For this review, take the finished solid that the model builds, in its own axes (mm). A direction names the side the tool comes from. Coordinates: 2 decimals unless noted, no trailing zeros. Loops run counter-clockwise (first coordinate to the right, second up) from the corner with the lowest first, then second, coordinate; pieces in that order, holes last.
1. Clearance check with flat-ended pins moving along their axes: P1, Ø4, axis at x = 7, z = 18.5, coming from the +Y side; P2, Ø4, axis at y = 8.5, z = 13, coming from the -X side; P3, Ø1, axis at y = 11, z = 27.5, coming from the -X side; P4, Ø12, axis at x = 0, y = 0, coming from the +Z side. State where each tip first meets the part, or that it passes through.
2. To check wall thickness, follow probe 1 along X at (y, z) = (0.5, 30); probe 2 along Y at (x, z) = (0, 9). State the ranges of each line that lie inside material, in increasing order.
3. Mouldability with a two-part tool opening along Y and no side actions: class faces 4 (the face through (0, -18.371, 27)), 5 (the face through (5, -7, 11.906)), 6 (the face through (8, -15, 21.828)) as pulls with the +Y half, pulls with the -Y half, needs draft (parallel to the pull), parting line crosses it, or undercut.
4. Take a section at A-A, the plane y = 0. State the section outline as (x, z) points.
5. Take a section at C-C, the plane z = 25.5. State the section outline as (x, y) points.
6. Machinability: for faces 1 (the face through (-3.62, -16.303, 10.761)), 2 (the face through (4.923, -9.464, 21.689)), 3 (the face through (12.91, -13.07, 26.72)), which of the approach directions +Z, -Z, +X, -X, +Y, -Y give a long, thin tool a straight path to every point of the face, cutting with its end or side? Answer none if there is none.
7. Take a section at D-D, the plane x = 15. State the section outline as (y, z) points, then the cut area to 3 significant figures.
```python
from build123d import *

# Parameters (mm, degrees)
OBJ1_R     = 10.668
OBJ1_DEPTH = 19.84375
OBJ2     = 7.6454
OBJ3 = 31.75
BOX001_W               = 36.7411
BOX001_H               = 36.7411
BOX001_DEPTH           = 9.921875
BOX001_PLACEMENT_ANGLE = 45
BOX_W                  = 36.7411
BOX_H                  = 36.7411
BOX_DEPTH              = 9.921875
OBJ4        = 16.7005
OBJ5    = 31.75


with BuildPart() as obj1:
    # obj1 → obj1 (new body)
    with BuildSketch(Plane.XY.offset(11.90625)):
        Circle(OBJ1_R)
    extrude(amount=OBJ1_DEPTH)


with BuildPart() as cone:
    # Cone → Cone (revolve)
    with BuildSketch(Plane.XZ):
        Polygon((0, 0), (12.17295, 0), (7.6454, 5.953125), (0, 5.953125), align=None)
    revolve(axis=Axis((0, 0, 0), (0, 0, 1)))


with BuildPart() as fusion001:
    with BuildSketch(Plane.XY):
        Circle(OBJ2)
    extrude(amount=OBJ3)

    # Fusion001: union obj1, Cone
    add(obj1.part)
    add(cone.part)


with BuildPart() as box001:
    # Box001 → Box001 (new body)
    with BuildSketch(Plane.XY):
        with Locations((18.37055, 18.37055)):
            Rectangle(BOX001_W, BOX001_H)
    extrude(amount=BOX001_DEPTH)


with BuildPart() as box001_1:
    # Box001 placement: moved
    add(box001.part.moved(Location((0, -25.979881, 0))).rotate(Axis((0, -25.979881, 0), (0, 0, 1)), BOX001_PLACEMENT_ANGLE))


with BuildPart() as common:
    # Box → Box (new body)
    with BuildSketch(Plane(origin=(-18.37055, -18.37055, 0), x_dir=(1, 0, 0), z_dir=(0, 0, 1))):
        with Locations((18.37055, 18.37055)):
            Rectangle(BOX_W, BOX_H)
    extrude(amount=BOX_DEPTH)

    # Common: intersect Box001
    add(box001_1.part, mode=Mode.INTERSECT)


with BuildPart() as common_1:
    # Common placement: moved
    add(common.part.moved(Location((0, 0, 21.828125))))


with BuildPart() as cut:
    with BuildSketch(Plane.XY):
        Circle(OBJ4)
    extrude(amount=OBJ5)

    # Fusion: union Common
    add(common_1.part)

    # Cut: cut Fusion001
    add(fusion001.part, mode=Mode.SUBTRACT)


solid = cut.part
```
Results list:
1. P1: stops at y = 15.93
1. P2: stops at x = -15.38
1. P3: stops at x = -15.48
1. P4: passes through
2. probe 1: x = -18.37 to -10.66, 10.66 to 18.37
2. probe 2: y = -16.7 to -7.65, 7.65 to 16.7
3. face 4: pulls with the -Y half
3. face 5: undercut
3. face 6: needs draft
4. outline: (-18.37, 21.83) - (-16.7, 21.83) - (-16.7, 0) - (-12.17, 0) - (-7.65, 5.95) - (-7.65, 11.91) - (-10.67, 11.91) - (-10.67, 31.75) - (-18.37, 31.75) - close; (7.65, 5.95) - (12.17, 0) - (16.7, 0) - (16.7, 21.83) - (18.37, 21.83) - (18.37, 31.75) - (10.67, 31.75) - (10.67, 11.91) - (7.65, 11.91) - close
5. outline: (-18.37, -7.61) - (-7.61, -18.37) - (7.61, -18.37) - (18.37, -7.61) - (18.37, 7.61) - (7.61, 18.37) - (-7.61, 18.37) - (-18.37, 7.61) - close; hole circle Ø21.34 at (0, 0)
6. face 1: -Z
6. face 2: +Z
6. face 3: +Z, -Z, +X, -Y
7. outline: (-10.98, 21.83) - (-7.34, 21.83) - (-7.34, 0) - (7.34, 0) - (7.34, 21.83) - (10.98, 21.83) - (10.98, 31.75) - (-10.98, 31.75) - close
7. area: 538 mm2
